Work out the finished part from the listing and answer in its coordinate system (mm). Face numbers are marked on the shaded views. Give positions to 0.01 mm unless a question says otherwise; leave off trailing zeros. Order: outer loops, then holes, each group sorted by start corner. A loop starts at its lowest first (then second) coordinate and runs counter-clockwise, first axis right, second up. Notation, with made-up numbers: (-32, 85) - (8, 85) arc R27 ccw to (8, 112) - close; hole circle Ø8 at (-25, 84). An arc over 180 degrees is marked (long way). Return JSON: item names as keys, results as strings. Group by question number.
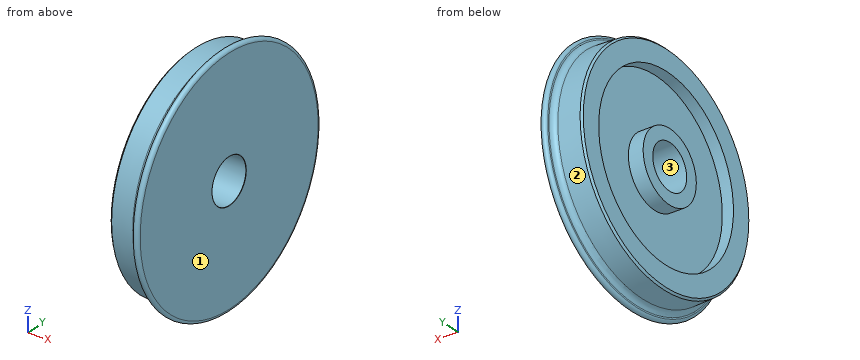
from build123d import *


with BuildPart() as part:
    # Sketch1 → Revolve1 (revolve)
    with BuildSketch(Plane.XY, mode=Mode.PRIVATE) as revolve1_sk:
        with BuildLine():
            Line((0, 20), (34.75, 20))
            ThreePointArc((34.75, 20), (34.926776695, 20.073223305), (35, 20.25))
            Line((35, 20.25), (35, 104.870611348))
            ThreePointArc((35, 104.870611348), (32.419685468, 107.661979883), (29.434472646, 105.308627851))
            Line((29.434472646, 105.308627851), (29.238441703, 104.070937185))
            ThreePointArc((29.238441703, 104.070937185), (27.613100241, 101.108330906), (24.474497484, 99.856155375))
            Line((24.474497484, 99.856155375), (4.957894968, 99.174620597))
            Line((4.957894968, 99.174620597), (3.3, 97.516725629))
            Line((3.3, 97.516725629), (3.3, 79.416725629))
            Line((3.3, 79.416725629), (13.3, 79.416725629))
            Line((13.3, 79.416725629), (13.3, 31.34))
            Line((13.3, 31.34), (0, 31.34))
            Line((0, 31.34), (0, 20))
        make_face()
    revolve(revolve1_sk.sketch.rotate(Axis((-146.164683843, 0, 0), (1, 0, 0)), 90), axis=Axis((-146.164683843, 0, 0), (1, 0, 0)))


solid = part.part
1. Consider probe 1 along Y at (x, z) = (11, 0); probe 2 along Y at (x, z) = (7, 0); probe 3 along X at (y, z) = (-55.5, -60.5). Determine where each line is inside the solid, lowest interval first. Write a range as from..to.
2. Determine the mould class of the marked faces 1, 2 and 3 for opening direction Y: released by +Y, released by -Y, zero draft, split by the parting line, or undercut.
3. The part is cut by section C-C (x = 19). Give the vertices of the cut face in (y, z).
4. The part is cut by section A-A (y = 0). Give the vertices of the cut face in (x, z).
5. Each of these flat-tipped pins is pushed along its axis until it touches: pin 1 (4 mm diameter, centred on x = 7.5, z = -84.5, fed in from +Y); pin 2 (1 mm diameter, centred on x = 27.5, y = -28, fed in from -Z); pin 3 (12 mm diameter, centred on x = 26.5, z = 76, fed in from -Y). Where does it stop, or does it pass through?
Answers:
{
 "1": {"probe 1": "y = -99.39..-79.42, -31.34..-20, 20..31.34, 79.42..99.39", "probe 2": "y = -99.25..-79.42, -31.34..-20, 20..31.34, 79.42..99.25", "probe 3": "x = 3.3..35"},
 "2": {"face 1": "zero draft", "face 2": "split by the parting line", "face 3": "undercut"},
 "3": {"outline": "circle Ø199.33 at (0, 0); hole circle Ø40 at (0, 0)"},
 "4": {"outline": "(0, -31.34) - (13.3, -31.34) - (13.3, -79.42) - (3.3, -79.42) - (3.3, -97.52) - (4.96, -99.17) - (24.47, -99.86) arc R5 cw to (29.24, -104.07) - (29.43, -105.31) arc R2.8 ccw to (35, -104.87) - (35, -20.25) arc R0.25 ccw to (34.75, -20) - (0, -20) - close; (0, 20) - (34.75, 20) arc R0.25 ccw to (35, 20.25) - (35, 104.87) arc R2.8 ccw to (29.43, 105.31) - (29.24, 104.07) arc R5 cw to (24.47, 99.86) - (4.96, 99.17) - (3.3, 97.52) - (3.3, 79.42) - (13.3, 79.42) - (13.3, 31.34) - (0, 31.34) - close"},
 "5": {"pin 1": "stops at y = 55.2", "pin 2": "stops at z = -97.57", "pin 3": "stops at y = -79.73"}
}
